The listing builds one solid part. Answer for the finished solid, in the listing's coordinates (mm). A direction names the side the tool comes from. Give positions to 0.01 mm unless a question says otherwise; leave off trailing zeros. Order: outer loops, then holes, each group sorted by start corner. A loop starts at its lowest first (then second) coordinate and runs counter-clockwise, first axis right, second up. Notation, with made-up numbers: (-20.75, 73) - (-15.75, 73) arc R14 cw to (-15.75, 77) - close; hole circle Ø8 at (14.25, 88). An arc over 180 degrees is marked (long way). Answer as a JSON object with one key per item and string values. Group by question number.
Q1. A cutting plane is placed at C-C, the plane y = 213. Give the vertices of the cut face in (x, z).
Q2. Given pin 1 (1.5 mm diameter, centred on x = 2, y = 203.5, fed in from +Z); pin 2 (1 mm diameter, centred on y = 230.5, z = -3, fed in from -X); pin 3 (3 mm diameter, centred on x = 0, z = 0, fed in from +Y), each flat-ended and moving along its own axis, determine where each tip first touches the part or whether it passes through.
Q3. A cutting plane is placed at A-A, the plane x = 0. Give the vertices of the cut face in (y, z).
Q4. The mould has two halves that part along Z. Classify faces 4 (the face through (2, 0, -2)), 5 (the face through (-0.867, 132.617, -3.905)), 6 (the face through (0, 257, 0)): released by +Z, released by -Z, zero draft, split by the parting line, or undercut.
Q5. A cutting plane is placed at B-B, the plane z = 0. Give the vertices of the cut face in (x, y), and give its area (3 significant figures).
Q6. Consider line 1 (Z direction, x = 0, y = 261.25); line 2 (Y direction, x = -0.5, z = 0.75); line 3 (X direction, y = 109, z = -0.5). Determine where each line is inside the solid, lowest interval first.
Q7. For faces 1 (the face through (2, 269, -2)), 2 (the face through (2.44, 263.08, 0.54)), 3 (the face through (-0.54, 5.92, -2.44)), determine the directions among +Z, -Z, +X, -X, +Y, -Y from which every point of the face is accessible in a straight line to the end or side of a thin tool.
Solid Edge part; units mm, degrees
sketch "Sketch1" plane through (0, 0, 0) normal (0, -1, 0) x (1, 0, 0)
  circle A0 centre (0, 0) radius 4
extrude "Protrusion1" add sketch "Sketch1" against normal blind 269
sketch "Sketch2" plane through (0, 269, 0) normal (0, 1, 0) x (0, 0, -1)
  circle A0 centre (0, 0) radius 2.5
extrude "ExtrudedCutout_2" cut sketch "Sketch2" against normal blind 12
sketch "Sketch3" plane through (0, 0, 0) normal (0, -1, 0) x (1, 0, 0)
  circle A0 centre (0, 0) radius 2.5
extrude "ExtrudedCutout_3" cut sketch "Sketch3" against normal blind 12
cosmetic_thread "Thread1"
cosmetic_thread "Thread2"
properties material "Steel"
Reply:
{
 "1": {"outline": "circle Ø8 at (0, 0)"},
 "2": {"pin 1": "stops at z = 3.8", "pin 2": "stops at x = -3.12", "pin 3": "stops at y = 257"},
 "3": {"outline": "(0, -4) - (269, -4) - (269, -2.5) - (257, -2.5) - (257, 2.5) - (269, 2.5) - (269, 4) - (0, 4) - (0, 2.5) - (12, 2.5) - (12, -2.5) - (0, -2.5) - close"},
 "4": {"face 4": "zero draft", "face 5": "split by the parting line", "face 6": "undercut"},
 "5": {"outline": "(-4, 0) - (-2.5, 0) - (-2.5, 12) - (2.5, 12) - (2.5, 0) - (4, 0) - (4, 269) - (2.5, 269) - (2.5, 257) - (-2.5, 257) - (-2.5, 269) - (-4, 269) - close", "area": "2,030 mm^2"},
 "6": {"line 1": "z = -4 to -2.5, 2.5 to 4", "line 2": "y = 12 to 257", "line 3": "x = -3.97 to 3.97"},
 "7": {"face 1": "+Z, -Z, +X, -X, +Y", "face 2": "+Y", "face 3": "-Y"}
}
